Geometry check sheet. Reference: the model listing, model coordinates, mm. A direction names the side the tool comes from. Give positions to 0.01 mm unless a question says otherwise; leave off trailing zeros. Write each loop counter-clockwise with the first axis right and the second up, starting at its lowest first coordinate (ties: lowest second). Pieces come first, ordered by that corner, then holes. Notation, with made-up numbers: (-26, 18) - (-18, 18) arc R6 ccw to (-18, 28) - close; hole circle Ø6 at (16, -27). An arc over 180 degrees is marked (long way). Use a Markdown table: item, result.
```python
from build123d import *

# Parameters (mm, degrees)
SKETCH_1_W          = 85
SKETCH_1_H          = 50
EXTRUDE_1_DEPTH     = 57
SKETCH_3_W          = 22
SKETCH_3_H          = 51
CUT_EXTRUDE_2_DEPTH = 82
CUT_EXTRUDE_4_REACH = 88.921
SKETCH_4_W          = 65
SKETCH_4_H          = 32


with BuildPart() as part:
    # 草图1 → 凸台-拉伸1 (new body)
    with BuildSketch(Plane(origin=(0, 0, 0), x_dir=(1, 0, 0), z_dir=(0, 1, 0))):
        Rectangle(SKETCH_1_W, SKETCH_1_H)
    extrude(amount=EXTRUDE_1_DEPTH)

    # 草图3 → 切除-拉伸2 (cut)
    with BuildSketch(Plane(origin=(42.5, 0, 0), x_dir=(0, 0, -1), z_dir=(1, 0, 0))):
        with Locations((-11, 28.5)):
            Rectangle(SKETCH_3_W, SKETCH_3_H)
        with Locations((11, 28.5)):
            Rectangle(SKETCH_3_W, SKETCH_3_H)
    extrude(amount=-CUT_EXTRUDE_2_DEPTH, mode=Mode.SUBTRACT)

    # 草图4 → 切除-拉伸4 (cut, up to next)
    with BuildSketch(Plane.XY.offset(25), mode=Mode.PRIVATE) as cut_extrude_4_sk1:
        with Locations((10, 28.5)):
            Rectangle(SKETCH_4_W, SKETCH_4_H)
    cut_extrude_4_tool1 = extrude(cut_extrude_4_sk1.sketch, amount=-CUT_EXTRUDE_4_REACH, mode=Mode.PRIVATE) & part.part
    add(cut_extrude_4_tool1.solids().sort_by_distance((10, 28.5, 25))[0], mode=Mode.SUBTRACT)


solid = part.part
```
1) Section check A-A on z = 3.5. Record the boundary of the cut face in (x, y), then the cut area to 3 significant figures.
Working result:
| item | result |
|---|---|
| outline | (-42.5, 0) - (42.5, 0) - (42.5, 3) - (-39.5, 3) - (-39.5, 54) - (42.5, 54) - (42.5, 57) - (-42.5, 57) - close |
| area | 663 mm² |
2) Material ranges on L1, parallel to Y at x = -13, z = -2.5; L2, parallel to Z at x = -33.5, y = 47; L3, parallel to X at y = 8, z = -5.5, recorded low to high. Write a range as from..to.
Working result:
| item | result |
|---|---|
| L1 | y = 0..3, 54..57 |
| L2 | z = -25..-22, 22..25 |
| L3 | x = -42.5..-39.5 |
3) Section check D-D on x = -9. Record the boundary of the cut face in (y, z), then the cut area to 3 significant figures.
Working result:
| item | result |
|---|---|
| outline | (0, -25) - (57, -25) - (57, 25) - (44.5, 25) - (44.5, 22) - (54, 22) - (54, -22) - (3, -22) - (3, 22) - (12.5, 22) - (12.5, 25) - (0, 25) - close |
| area | 510 mm² |
4) Section check C-C on x = -29. Record the boundary of the cut face in (y, z).
Working result:
| item | result |
|---|---|
| outline | (0, -25) - (57, -25) - (57, 25) - (0, 25) - close; hole (3, -22) - (54, -22) - (54, 22) - (3, 22) - close |
5) Set-up check for faces 4 (the flat face through (-1, 28, -25)), 5 (the flat face through (-7, 45, 22)), 6 (the flat face through (10, 12.5, 24)): record each of +Z, -Z, +X, -X, +Y, -Y from which the full face is reachable in a straight line by a thin tool's end or side.
Working result:
| item | result |
|---|---|
| face 4 | -Z, +X, -X, +Y, -Y |
| face 5 | +X |
| face 6 | +Z, +X |
6) Depth check by flat-ended pin: P1, Ø2.5, axis at y = 34.5, z = 23.5, coming from the +X side; P2, Ø10, axis at x = 9.5, y = 33, coming from the +Z side. Enter the tip coordinate at first touch or a pass-through.
Working result:
| item | result |
|---|---|
| P1 | stops at x = -22.5 |
| P2 | stops at z = -22 |
7) Mould release check, pull along Y, two halves, no side actions. Record for faces 1 (the flat face through (10, 44.5, 24)), 2 (the flat face through (-10, 9, 25)), 3 (the flat face through (-1, 57, 0)): pulls with the +Y half, pulls with the -Y half, needs draft (parallel to the pull), parting line crosses it, or undercut.
Working result:
| item | result |
|---|---|
| face 1 | undercut |
| face 2 | needs draft |
| face 3 | pulls with the +Y half |
8) Section check B-B on y = 51. Record the boundary of the cut face in (x, z).
Working result:
| item | result |
|---|---|
| outline | (-42.5, -25) - (42.5, -25) - (42.5, -22) - (-39.5, -22) - (-39.5, 22) - (42.5, 22) - (42.5, 25) - (-42.5, 25) - close |
